Here's how the part is built. I have some questions about the finished solid (model axes, mm). A direction names the side the tool comes from. Coordinates: 2 decimals unless noted, no trailing zeros. Write each loop counter-clockwise with the first axis right and the second up, starting at its lowest first coordinate (ties: lowest second). Pieces come first, ordered by that corner, then holes.
from build123d import *

# Parameters (mm, degrees)
SM_BASE_FLANGE_1_DEPTH            = 2
SM_EDGE_FLANGE_1_STRIP_W          = 12
SM_EDGE_FLANGE_1_STRIP_H          = 2
SM_EDGE_FLANGE_1_STRIP_CUT_DEPTH  = 50
SM_EDGE_FLANGE_1_RELIEF_W         = 13
SM_EDGE_FLANGE_1_RELIEF_H         = 1
SM_EDGE_FLANGE_1_RELIEF_CUT_DEPTH = 2
SM_EDGE_FLANGE_1_DEPTH            = 50
SM_EDGE_FLANGE_2_STRIP_W          = 12
SM_EDGE_FLANGE_2_STRIP_H          = 2
SM_EDGE_FLANGE_2_STRIP_CUT_DEPTH  = 50
SM_EDGE_FLANGE_2_RELIEF_W         = 13
SM_EDGE_FLANGE_2_RELIEF_H         = 1
SM_EDGE_FLANGE_2_RELIEF_CUT_DEPTH = 2
SM_EDGE_FLANGE_2_DEPTH            = 50
SM_EDGE_FLANGE_3_STRIP_W          = 13
SM_EDGE_FLANGE_3_STRIP_H          = 2
SM_EDGE_FLANGE_3_STRIP_CUT_DEPTH  = 36
SM_EDGE_FLANGE_3_RELIEF_W         = 14
SM_EDGE_FLANGE_3_RELIEF_H         = 1
SM_EDGE_FLANGE_3_RELIEF_CUT_DEPTH = 2
SM_EDGE_FLANGE_3_DEPTH            = 36
SM_EDGE_FLANGE_4_STRIP_W          = 13
SM_EDGE_FLANGE_4_STRIP_H          = 2
SM_EDGE_FLANGE_4_STRIP_CUT_DEPTH  = 36
SM_EDGE_FLANGE_4_RELIEF_W         = 14
SM_EDGE_FLANGE_4_RELIEF_H         = 1
SM_EDGE_FLANGE_4_RELIEF_CUT_DEPTH = 2
SM_EDGE_FLANGE_4_DEPTH            = 36
CHAMFER_1_SIZE                    = 5
HOLE_WIZARD_M61_AT_2_COUNT        = 2
HOLE_WIZARD_M61_AT_2_PITCH        = 18
HOLE_WIZARD_M61_AT_3_COUNT        = 2
HOLE_WIZARD_M61_AT_3_PITCH        = 325
HOLE_WIZARD_M61_AT_4_COUNT        = 2
HOLE_WIZARD_M61_AT_4_PITCH        = 343
SKETCH_20_R                       = 2.5
CUT_EXTRUDE_1_DEPTH               = 2
SKETCH_21_W                       = 645
SKETCH_21_H                       = 2
CUT_EXTRUDE_2_DEPTH               = 2


# Sheet-metal steps are written as plain solids
with BuildPart() as part:
    # Sketch 1 → Базовая кромка1 (new body)
    with BuildSketch(Plane(origin=(0, 0, 0), x_dir=(1, 0, 0), z_dir=(0, 1, 0))):
        with BuildLine():
            Line((-187.5, 0), (187.5, 0))
            ThreePointArc((187.5, 0), (189.588419076, 0.136882218), (191.641104722, 0.545186779))
            Line((191.641104722, 0.545186779), (361.641104722, 46.096549493))
            ThreePointArc((361.641104722, 46.096549493), (370.193653445, 51.811179849), (373.5, 61.551362713))
            Line((373.5, 61.551362713), (373.5, 84))
            Line((373.5, 84), (0, 84))
            Line((0, 84), (-373.5, 84))
            Line((-373.5, 84), (-373.5, 61.551362713))
            ThreePointArc((-373.5, 61.551362713), (-370.193653445, 51.811179849), (-361.641104722, 46.096549493))
            Line((-361.641104722, 46.096549493), (-191.641104722, 0.545186779))
            ThreePointArc((-191.641104722, 0.545186779), (-189.588419076, 0.136882218), (-187.5, 0))
        make_face()
    extrude(amount=SM_BASE_FLANGE_1_DEPTH)

    # Ребро-кромка1 strip (across the edge) → Ребро-кромка1 strip cut (cut)
    with BuildSketch(Plane(origin=(323.5, 0, -84), x_dir=(0, 0, 1), z_dir=(1, 0, 0))):
        with Locations((-2, -1)):
            Rectangle(SM_EDGE_FLANGE_1_STRIP_W, SM_EDGE_FLANGE_1_STRIP_H)
    extrude(amount=SM_EDGE_FLANGE_1_STRIP_CUT_DEPTH, mode=Mode.SUBTRACT)

    # Ребро-кромка1 relief (on the sheet) → Ребро-кромка1 relief cut (cut)
    with BuildSketch(Plane(origin=(323.5, 0, -80), x_dir=(0, 0, 1), z_dir=(0, -1, 0))):
        with Locations((-5.5, 0.5)):
            Rectangle(SM_EDGE_FLANGE_1_RELIEF_W, SM_EDGE_FLANGE_1_RELIEF_H)
    extrude(amount=-SM_EDGE_FLANGE_1_RELIEF_CUT_DEPTH, mode=Mode.SUBTRACT)

    # Ребро-кромка1 section (across the edge) → Ребро-кромка1 (add)
    with BuildSketch(Plane(origin=(323.5, 0, -84), x_dir=(0, 0, 1), z_dir=(1, 0, 0))):
        with BuildLine():
            Line((0, 2), (0, 25))
            Line((0, 25), (2, 25))
            Line((2, 25), (2, 2))
            ThreePointArc((2, 2), (2.585786438, 0.585786438), (4, 0))
            Line((4, 0), (4, -2))
            ThreePointArc((4, -2), (1.171572875, -0.828427125), (0, 2))
        make_face()
    extrude(amount=SM_EDGE_FLANGE_1_DEPTH)

    # Ребро-кромка2 strip (across the edge) → Ребро-кромка2 strip cut (cut)
    with BuildSketch(Plane(origin=(-373.5, 0, -84), x_dir=(0, 0, 1), z_dir=(1, 0, 0))):
        with Locations((-2, -1)):
            Rectangle(SM_EDGE_FLANGE_2_STRIP_W, SM_EDGE_FLANGE_2_STRIP_H)
    extrude(amount=SM_EDGE_FLANGE_2_STRIP_CUT_DEPTH, mode=Mode.SUBTRACT)

    # Ребро-кромка2 relief (on the sheet) → Ребро-кромка2 relief cut (cut)
    with BuildSketch(Plane(origin=(-373.5, 0, -80), x_dir=(0, 0, 1), z_dir=(0, -1, 0))):
        with Locations((-5.5, -50.5)):
            Rectangle(SM_EDGE_FLANGE_2_RELIEF_W, SM_EDGE_FLANGE_2_RELIEF_H)
    extrude(amount=-SM_EDGE_FLANGE_2_RELIEF_CUT_DEPTH, mode=Mode.SUBTRACT)

    # Ребро-кромка2 section (across the edge) → Ребро-кромка2 (add)
    with BuildSketch(Plane(origin=(-373.5, 0, -84), x_dir=(0, 0, 1), z_dir=(1, 0, 0))):
        with BuildLine():
            Line((0, 2), (0, 25))
            Line((0, 25), (2, 25))
            Line((2, 25), (2, 2))
            ThreePointArc((2, 2), (2.585786438, 0.585786438), (4, 0))
            Line((4, 0), (4, -2))
            ThreePointArc((4, -2), (1.171572875, -0.828427125), (0, 2))
        make_face()
    extrude(amount=SM_EDGE_FLANGE_2_DEPTH)

    # Ребро-кромка3 strip (across the edge) → Ребро-кромка3 strip cut (cut)
    with BuildSketch(Plane(origin=(-144.5, 0, 1), x_dir=(0, 0, -1), z_dir=(-1, 0, 0))):
        with Locations((-2.5, -1)):
            Rectangle(SM_EDGE_FLANGE_3_STRIP_W, SM_EDGE_FLANGE_3_STRIP_H)
    extrude(amount=SM_EDGE_FLANGE_3_STRIP_CUT_DEPTH, mode=Mode.SUBTRACT)

    # Ребро-кромка3 relief (on the sheet) → Ребро-кромка3 relief cut (cut)
    with BuildSketch(Plane(origin=(-144.5, 0, -3), x_dir=(0, 0, -1), z_dir=(0, -1, 0))):
        with Locations((-6, 0.5)):
            Rectangle(SM_EDGE_FLANGE_3_RELIEF_W, SM_EDGE_FLANGE_3_RELIEF_H)
        with Locations((-6, -36.5)):
            Rectangle(SM_EDGE_FLANGE_3_RELIEF_W, SM_EDGE_FLANGE_3_RELIEF_H)
    extrude(amount=-SM_EDGE_FLANGE_3_RELIEF_CUT_DEPTH, mode=Mode.SUBTRACT)

    # Ребро-кромка3 section (across the edge) → Ребро-кромка3 (add)
    with BuildSketch(Plane(origin=(-144.5, 0, 1), x_dir=(0, 0, -1), z_dir=(-1, 0, 0))):
        with BuildLine():
            Line((0, 2), (0, 25))
            Line((0, 25), (2, 25))
            Line((2, 25), (2, 2))
            ThreePointArc((2, 2), (2.585786438, 0.585786438), (4, 0))
            Line((4, 0), (4, -2))
            ThreePointArc((4, -2), (1.171572875, -0.828427125), (0, 2))
        make_face()
    extrude(amount=SM_EDGE_FLANGE_3_DEPTH)

    # Ребро-кромка4 strip (across the edge) → Ребро-кромка4 strip cut (cut)
    with BuildSketch(Plane(origin=(180.5, 0, 1), x_dir=(0, 0, -1), z_dir=(-1, 0, 0))):
        with Locations((-2.5, -1)):
            Rectangle(SM_EDGE_FLANGE_4_STRIP_W, SM_EDGE_FLANGE_4_STRIP_H)
    extrude(amount=SM_EDGE_FLANGE_4_STRIP_CUT_DEPTH, mode=Mode.SUBTRACT)

    # Ребро-кромка4 relief (on the sheet) → Ребро-кромка4 relief cut (cut)
    with BuildSketch(Plane(origin=(180.5, 0, -3), x_dir=(0, 0, -1), z_dir=(0, -1, 0))):
        with Locations((-6, 0.5)):
            Rectangle(SM_EDGE_FLANGE_4_RELIEF_W, SM_EDGE_FLANGE_4_RELIEF_H)
        with Locations((-6, -36.5)):
            Rectangle(SM_EDGE_FLANGE_4_RELIEF_W, SM_EDGE_FLANGE_4_RELIEF_H)
    extrude(amount=-SM_EDGE_FLANGE_4_RELIEF_CUT_DEPTH, mode=Mode.SUBTRACT)

    # Ребро-кромка4 section (across the edge) → Ребро-кромка4 (add)
    with BuildSketch(Plane(origin=(180.5, 0, 1), x_dir=(0, 0, -1), z_dir=(-1, 0, 0))):
        with BuildLine():
            Line((0, 2), (0, 25))
            Line((0, 25), (2, 25))
            Line((2, 25), (2, 2))
            ThreePointArc((2, 2), (2.585786438, 0.585786438), (4, 0))
            Line((4, 0), (4, -2))
            ThreePointArc((4, -2), (1.171572875, -0.828427125), (0, 2))
        make_face()
    extrude(amount=SM_EDGE_FLANGE_4_DEPTH)

    # Фаска1
    chamfer_1_edges = [part.edges().sort_by_distance(p)[0] for p in [
        (-373.5, -25, -83),
        (-323.5, -25, -83),
        (-144.5, -25, 0),
        (-180.5, -25, 0),
        (180.5, -25, 0),
        (144.5, -25, 0),
        (323.5, -25, -83),
        (373.5, -25, -83),
    ]]
    chamfer(chamfer_1_edges, length=CHAMFER_1_SIZE)

    # Эскиз18 → Зенковка для винта с потайной головкой M61 (revolve, cut)
    with BuildSketch(Plane(origin=(-171.5, -11, 1), x_dir=(0, -1, 0), z_dir=(1, 0, 0))):
        Polygon((0, 0), (0, 2), (4.5, 2), (4.5, 1.5), (6, 0), align=None)
    hole_wizard_m61 = revolve(axis=Axis((-171.5, -11, 7.35), (0, 0, -1)), mode=Mode.SUBTRACT)

    # Зенковка для винта с потайной головкой M61 at 2: Зенковка для винта с потайной головкой M61 ×2
    with Locations(*[(i * HOLE_WIZARD_M61_AT_2_PITCH, 0, 0) for i in range(1, HOLE_WIZARD_M61_AT_2_COUNT)]):
        add(hole_wizard_m61, mode=Mode.SUBTRACT)

    # Зенковка для винта с потайной головкой M61 at 3: Зенковка для винта с потайной головкой M61 ×2
    with Locations(*[(i * HOLE_WIZARD_M61_AT_3_PITCH, 0, 0) for i in range(1, HOLE_WIZARD_M61_AT_3_COUNT)]):
        add(hole_wizard_m61, mode=Mode.SUBTRACT)

    # Зенковка для винта с потайной головкой M61 at 4: Зенковка для винта с потайной головкой M61 ×2
    with Locations(*[(i * HOLE_WIZARD_M61_AT_4_PITCH, 0, 0) for i in range(1, HOLE_WIZARD_M61_AT_4_COUNT)]):
        add(hole_wizard_m61, mode=Mode.SUBTRACT)

    # Эскиз20 → Вытянуть1 (cut)
    with BuildSketch(Plane(origin=(0, 0, -84), x_dir=(-1, 0, 0), z_dir=(0, 0, -1))):
        with Locations(Location((337.5, -11, 0), (0, 0, 90))):
            Circle(SKETCH_20_R)
        with Locations(Location((359.5, -11, 0), (0, 0, 90))):
            Circle(SKETCH_20_R)
        with Locations(Location((-359.5, -11, 0), (0, 0, 270))):
            Circle(SKETCH_20_R)
        with Locations(Location((-337.5, -11, 0), (0, 0, 270))):
            Circle(SKETCH_20_R)
    extrude(amount=-CUT_EXTRUDE_1_DEPTH, mode=Mode.SUBTRACT)

    # Эскиз21 → Вытянуть2 (cut)
    with BuildSketch(Plane(origin=(0, 0, -84), x_dir=(-1, 0, 0), z_dir=(0, 0, -1))):
        with Locations((0, 1)):
            Rectangle(SKETCH_21_W, SKETCH_21_H)
    extrude(amount=-CUT_EXTRUDE_2_DEPTH, mode=Mode.SUBTRACT)


solid = part.part
1. If I drill on line 1 (Y direction, x = 359.5, z = -82.5); line 2 (Y direction, x = 2, z = -60.5); line 3 (Z direction, x = 52, y = 1), over which ranges is the centre line in solid material (lowest first)?
2. For pin 1 Ø6.5 at (x, y) = (359.5, -11) entering from +Z; pin 2 Ø7 at (x, y) = (166.5, -15.5) entering from -Z; pin 3 Ø1.5 at (y, z) = (-10.5, -81) entering from +X; pin 4 Ø12 at (x, y) = (-292, -1) entering from -Z, each with a flat end and sliding along its axis, tell me the tip position at first contact or that it passes through.
3. On a 3-axis mill with a long thin cutter (end or side, diameter ignored), from which of +Z, -Z, +X, -X, +Y, -Y can I reach the whole of each face in a straight line? I mean faces 1 (the face through (-162, -14, -1)), 2 (the face through (-373.5, 1, -78)), 3 (the face through (348, -14, -82)). Say none if no direction works.
4. I want a section at A-A (z = -69.5). List the corners of the cut face in (x, y) for me.
5. I want a section at B-B (x = -110). List the corners of the cut face in (y, z) for me.
Response values:
1. line 1: y = -25 to -13.5, -8.5 to 1.12
1. line 2: y = 0 to 2
1. line 3: z = -82 to 0
2. pin 1: stops at z = -82
2. pin 2: stops at z = -1
2. pin 3: passes through
2. pin 4: stops at z = -82
3. face 1: -Z, +X, -X, -Y
3. face 2: +Z, -Z, -X, +Y, -Y
3. face 3: +Z, +X, -X, -Y
4. outline: (-373.5, 0) - (373.5, 0) - (373.5, 2) - (-373.5, 2) - close
5. outline: (0, -82) - (2, -82) - (2, 0) - (0, 0) - close
